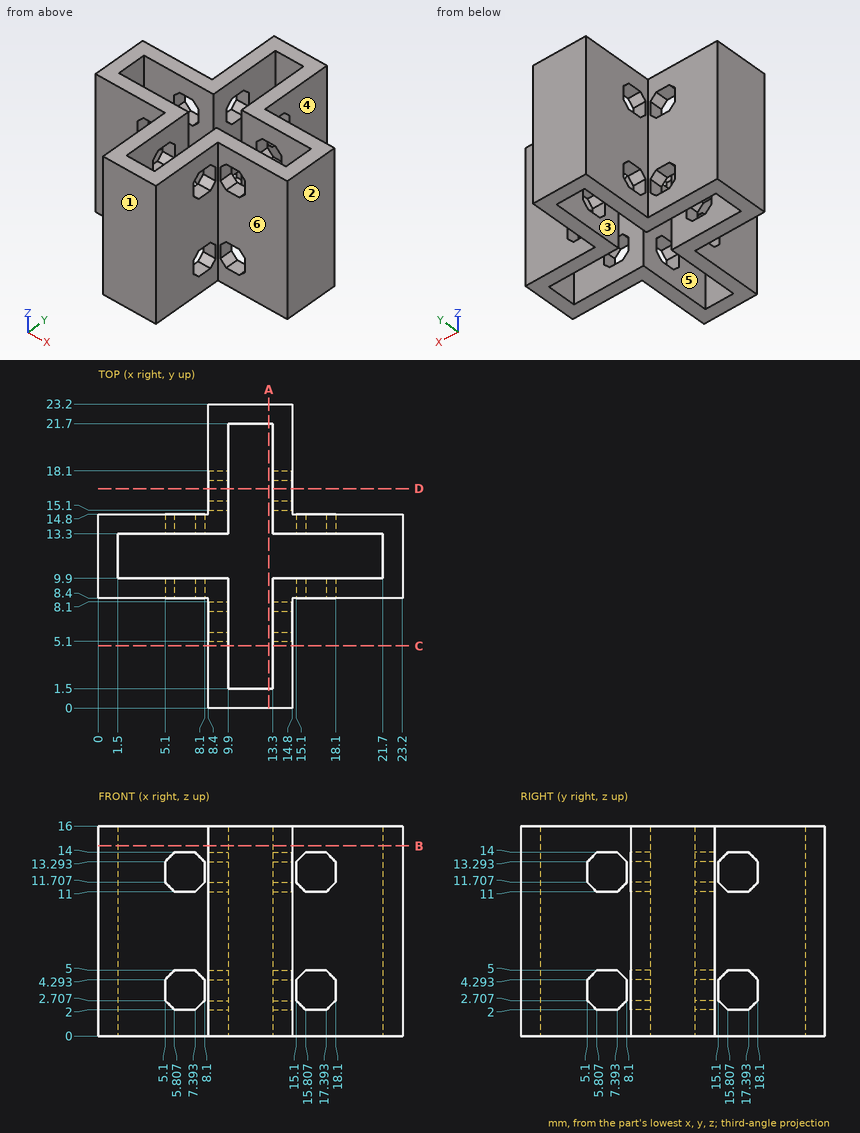
Study the drawing (mm; zero at the part's minimum x, y, z) and answer. A direction names the side the tool comes from. Give positions to 0.01 mm unless a question says otherwise; leave off trailing zeros. Loops run counter-clockwise (first coordinate to the right, second up) from the corner with the lowest first, then second, coordinate; pieces in that order, holes last. Notation, with made-up numbers: (47, -2.5) -> (95, -2.5) arc R20 cw to (95, 26.5) -> close; hole circle Ø8 at (61, 49). An arc over 180 degrees is marked (long way). Use a Markdown table: item, result. Add a question column.
1) Which of the six approach directions +Z, -Z, +X, -X, +Y, -Y give full straight-line access (tool end or side, diameter ignored) to the marked faces 4, 5 and 6?
2) The part is cut by section D-D, the plane y = 16.75. Determine the outline of the cut face in (x, z), plus the area to 3 significant figures.
3) For a pull along X with two mould halves and no side action, classify the marked faces 1, 2 and 3 as +X half, -X half, draft (parallel to the pull), parting line (faces both ways), or undercut.
4) The part is cut by section B-B, the plane z = 14.5. Determine the outline of the cut face in (x, y), plus the area to 3 significant figures.
5) Consider line 1 along X through (y, z) = (4, 2.75); line 2 along Y through (x, z) = (14, 7.5). Determine where each line is inside the solid, lowest interval first.
6) Each of these flat-tipped pins is pushed along its axis until it touches: P1, Ø4, axis at x = 5.5, z = 10.5, coming from the +Y side; P2, Ø1.5, axis at y = 20, z = 9, coming from the +X side; P3, Ø6, axis at y = 18, z = 10.5, coming from the -X side. Where does it stop, or does it pass through?
7) The part is cut by section A-A, the plane x = 13. Determine the outline of the cut face in (y, z), plus the area to 3 significant figures.
8) The part is cut by section C-C, the plane y = 4.75. Determine the outline of the cut face in (x, z).
Reported:
| question | item | result |
|---|---|---|
| 1 | face 4 | +Z, -Z, +X, +Y |
| 1 | face 5 | +Z, -Z |
| 1 | face 6 | +Z, -Z, +X, -Y |
| 2 | outline | (8.4, 0) -> (9.9, 0) -> (9.9, 2) -> (8.4, 2) -> close; (8.4, 5) -> (9.9, 5) -> (9.9, 11) -> (8.4, 11) -> close; (8.4, 14) -> (9.9, 14) -> (9.9, 16) -> (8.4, 16) -> close; (13.3, 0) -> (14.8, 0) -> (14.8, 2) -> (13.3, 2) -> close; (13.3, 5) -> (14.8, 5) -> (14.8, 11) -> (13.3, 11) -> close; (13.3, 14) -> (14.8, 14) -> (14.8, 16) -> (13.3, 16) -> close |
| 2 | area | 30.0 mm^2 |
| 3 | face 1 | draft |
| 3 | face 2 | +X half |
| 3 | face 3 | undercut |
| 4 | outline | (0, 8.4) -> (8.4, 8.4) -> (8.4, 0) -> (14.8, 0) -> (14.8, 8.4) -> (23.2, 8.4) -> (23.2, 14.8) -> (14.8, 14.8) -> (14.8, 23.2) -> (8.4, 23.2) -> (8.4, 14.8) -> (0, 14.8) -> close; hole (1.5, 9.9) -> (9.9, 9.9) -> (9.9, 1.5) -> (13.3, 1.5) -> (13.3, 9.9) -> (21.7, 9.9) -> (21.7, 13.3) -> (13.3, 13.3) -> (13.3, 21.7) -> (9.9, 21.7) -> (9.9, 13.3) -> (1.5, 13.3) -> close |
| 4 | area | 130 mm^2 |
| 5 | line 1 | x = 8.4 to 9.9, 13.3 to 14.8 |
| 5 | line 2 | y = 0 to 9.9, 13.3 to 23.2 |
| 6 | P1 | stops at y = 14.8 |
| 6 | P2 | stops at x = 14.8 |
| 6 | P3 | stops at x = 8.4 |
| 7 | outline | (0, 0) -> (1.5, 0) -> (1.5, 16) -> (0, 16) -> close; (21.7, 0) -> (23.2, 0) -> (23.2, 16) -> (21.7, 16) -> close |
| 7 | area | 48.0 mm^2 |
| 8 | outline | (8.4, 0) -> (9.9, 0) -> (9.9, 16) -> (8.4, 16) -> close; (13.3, 0) -> (14.8, 0) -> (14.8, 16) -> (13.3, 16) -> close |
